CAD build for the part. Positions are in the model's coordinates, mm. A direction names the side the tool comes from. Coordinates: 2 decimals unless noted, no trailing zeros. Order: outer loops, then holes, each group sorted by start corner. A loop starts at its lowest first (then second) coordinate and runs counter-clockwise, first axis right, second up.
from build123d import *

# Parameters (mm, degrees)
SKETCH1_R           = 1.4605
BOSS_EXTRUDE1_DEPTH = 12.7
BOSS_EXTRUDE2_DEPTH = 14.2748
FILLET1_R           = 12.7
SKETCH3_R           = 3.2639
CUT_EXTRUDE1_DEPTH  = 89.397576146


with BuildPart() as part:
    # Sketch1 → Boss-Extrude1 (new body)
    with BuildSketch(Plane(origin=(0, 0, 0), x_dir=(1, 0, 0), z_dir=(0, 1, 0))):
        Polygon((-12.7, -23.622), (12.7, -23.622), (19.05, -23.622), (19.05, 23.622), (12.7, 23.622), (-12.7, 23.622), align=None)
        with Locations(Location((0, 12.7, 0), (0, 0, 270))):
            Circle(SKETCH1_R, mode=Mode.SUBTRACT)
        with Locations(Location((0, -12.7, 0), (0, 0, 270))):
            Circle(SKETCH1_R, mode=Mode.SUBTRACT)
    extrude(amount=BOSS_EXTRUDE1_DEPTH)

    # Sketch2 → Boss-Extrude2 (add)
    with BuildSketch(Plane(origin=(19.05, 0, 0), x_dir=(0, 0, -1), z_dir=(1, 0, 0))):
        Polygon((-23.622, 0), (-23.622, -50.546), (23.622, -50.546), (23.622, 71.6788), (-23.622, 71.6788), align=None)
    extrude(amount=BOSS_EXTRUDE2_DEPTH)

    # Fillet1
    fillet1_edges = [part.edges().sort_by_distance(p)[0] for p in [
        (19.05, 12.7, 0),
        (19.05, 0, 0),
    ]]
    fillet(fillet1_edges, radius=FILLET1_R)

    # Sketch3 → Cut-Extrude1 (cut, through all)
    with BuildSketch(Plane(origin=(33.3248, 0, 0), x_dir=(0, 0, -1), z_dir=(1, 0, 0))):
        with Locations((-12.7, -39.0398)):
            Circle(SKETCH3_R)
        with Locations((12.7, -39.0398)):
            Circle(SKETCH3_R)
        with Locations((-12.7, 59.3852)):
            Circle(SKETCH3_R)
        with Locations((12.7, 59.3852)):
            Circle(SKETCH3_R)
    extrude(amount=-CUT_EXTRUDE1_DEPTH, mode=Mode.SUBTRACT)


solid = part.part
1) Drill centre lines: probe 1 along Y at (x, z) = (23, -12.7); probe 2 along X at (y, z) = (3, -12.7); probe 3 along Y at (x, z) = (26, 14). Where is each one in solid material? Low to high.
2) Slice it at A-A (z = -12.7). List the corners of the cut face in (x, y).
3) Slice it at D-D (y = 33). List the corners of the cut face in (x, z).
4) Two-plate mould, pull along Z, no slides. Class faces 1 (the flat face through (19.05, 49, 0)), 2 (the flat face through (20, 11, 23.622)), 3 (the cylindrical face through (0.06, 6.26, -14.16)): released by +Z, released by -Z, zero draft, split by the parting line, or undercut.
5) Pin check, flat tips, straight feed: P1, Ø15, axis at x = -5, z = 9.5, coming from the -Y side; P2, Ø12, axis at x = 9, z = 19, coming from the -Y side; P3, Ø9.5, axis at x = -0.5, z = 5.5, coming from the +Y side. Stop position of each tip, or through.
6) Slice it at C-C (z = 17.5). List the corners of the cut face in (x, y), plus the area to 3 significant figures.
7) Which spindle directions (+Z, -Z, +X, -X, +Y, -Y) get a long thin tool onto all of the face, cutting with end or side? Do faces 4 (the flat face through (-3, 0, 0)), 5 (the flat face through (-3, 12.7, 0)), 6 (the cylindrical face through (0.06, 6.26, 11.24)). Say none if no direction does.
8) Slice it at B-B (x = 0). List the corners of the cut face in (y, z).
Worked out:
1. probe 1: y = -50.55 to -42.3, -35.78 to 56.12, 62.65 to 71.68
1. probe 2: x = -12.7 to -1.46, 1.46 to 33.32
1. probe 3: y = -50.55 to -42.03, -36.05 to 56.39, 62.38 to 71.68
2. outline: (-12.7, 0) - (-1.46, 0) - (-1.46, 12.7) - (-12.7, 12.7) - close; (1.46, 0) - (6.35, 0) arc R12.7 cw to (19.05, -12.7) - (19.05, -35.78) - (33.32, -35.78) - (33.32, 56.12) - (19.05, 56.12) - (19.05, 25.4) arc R12.7 cw to (6.35, 12.7) - (1.46, 12.7) - close; (19.05, -50.55) - (33.32, -50.55) - (33.32, -42.3) - (19.05, -42.3) - close; (19.05, 62.65) - (33.32, 62.65) - (33.32, 71.68) - (19.05, 71.68) - close
3. outline: (19.05, -23.62) - (33.32, -23.62) - (33.32, 23.62) - (19.05, 23.62) - close
4. face 1: zero draft
4. face 2: released by +Z
4. face 3: undercut
5. P1: stops at y = 0
5. P2: stops at y = -3.4
5. P3: stops at y = 12.7
6. outline: (-12.7, 0) - (6.35, 0) arc R12.7 cw to (19.05, -12.7) - (19.05, -50.55) - (33.32, -50.55) - (33.32, 71.68) - (19.05, 71.68) - (19.05, 25.4) arc R12.7 cw to (6.35, 12.7) - (-12.7, 12.7) - close
6. area: 2,220 mm2
7. face 4: +Z, -Z, -X, -Y
7. face 5: +Z, -Z, -X, +Y
7. face 6: +Y, -Y
8. outline: (0, -23.62) - (12.7, -23.62) - (12.7, -14.16) - (0, -14.16) - close; (0, -11.24) - (12.7, -11.24) - (12.7, 11.24) - (0, 11.24) - close; (0, 14.16) - (12.7, 14.16) - (12.7, 23.62) - (0, 23.62) - close
